Part model, mm, in its own coordinate system. Face numbers are marked on the shaded views. A direction names the side the tool comes from. Round coordinates to 2 decimals unless told otherwise and drop trailing zeros. Write each loop counter-clockwise with the first axis right and the second up, starting at its lowest first coordinate (ties: lowest second). Pieces come first, ordered by that corner, then holes. Notation, with made-up numbers: M -26,38 L 5,38 A29 ccw 5,67 Z; hole C -17.75,-2.5 d3. An arc over 180 degrees is marked long. Answer as a JSON object with one key per item and string values. Group by question number.
1. Two-plate mould, pull along X, no slides. Class the marked faces 1, 2 and 3: +X half, -X half, draft (parallel to the pull), parting line (faces both ways), or undercut.
2. Drop flat-ended pins along their axis: pin 1 (5 mm diameter, centred on y = 8, z = 6, fed in from +X); pin 2 (1.4 mm diameter, centred on x = -7, z = 15, fed in from +Y); pin 3 (1.8 mm diameter, centred on y = 11, z = 7.5, fed in from +X). Give the stop position or say it passes through.
3. Drill centre lines: line 1 (Z direction, x = -7.5, y = 2.55); line 2 (X direction, y = 5.25, z = 1.5); line 3 (Y direction, x = 5.75, z = 18.5). Where is each one in solid material? Low to high. Write a range as from..to.
4. Band-saw the part on D-D, the plane z = 16.25. Write the cut outline in (x, y).
5. Which spindle directions (+Z, -Z, +X, -X, +Y, -Y) get a long thin tool onto all of the face, cutting with end or side? Do the marked faces 4, 5 and 6. Say none if no direction does.
6. Band-saw the part on B-B, the plane z = 10. Write the cut outline in (x, y), plus the area to 3 significant figures.
7. Band-saw the part on C-C, the plane y = 2.5. Write the cut outline in (x, z), plus the area to 3 significant figures.
8. Band-saw the part on A-A, the plane x = -7.5. Write the cut outline in (y, z), plus the area to 3 significant figures.
from build123d import *

# Parameters (mm, degrees)
MAIN_DEPTH         = 20
SKETCH1_R          = 1.6
CUT_EXTRUDE1_DEPTH = 14


with BuildPart() as part:
    # Esquisse1 → Main (new body)
    with BuildSketch(Plane.XY):
        Polygon((-12.5, 0), (-12.5, 3), (-8.95, 3), (-8.95, 4), (-6.05, 4), (-6.05, 3), (-2.5, 3), (-2.5, 6.55), (-3.5, 6.55), (-3.5, 9.45), (-2.5, 9.45), (-2.5, 13), (0, 13), (0, 0), align=None)
    main = extrude(amount=MAIN_DEPTH)

    # Symétrie1: Main across plane
    add(main.mirror(Plane(origin=(0, 0, 0), x_dir=(0, 0, 1), z_dir=(1, 0, 0))))

    # Sketch1 → Cut-Extrude1 (cut, through all)
    with BuildSketch(Plane.XZ):
        with Locations((-7.5, 10)):
            Circle(SKETCH1_R)
        with Locations((7.5, 10)):
            Circle(SKETCH1_R)
    extrude(amount=-CUT_EXTRUDE1_DEPTH, mode=Mode.SUBTRACT)


solid = part.part
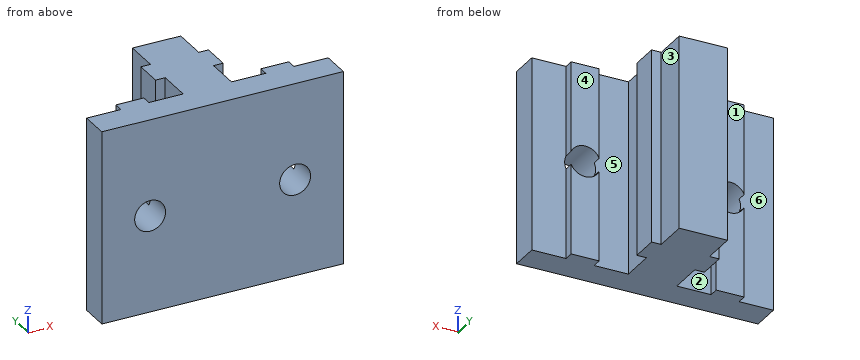
Worked answers:
{
 "1": {"face 1": "draft", "face 2": "undercut", "face 3": "+X half"},
 "2": {"pin 1": "stops at x = 3.5", "pin 2": "stops at y = 4", "pin 3": "stops at x = 2.5"},
 "3": {"line 1": "z = 0..8.4, 11.6..20", "line 2": "x = -2.5..2.5", "line 3": "y = 0..3"},
 "4": {"outline": "M -12.5,0 L 12.5,0 L 12.5,3 L 8.95,3 L 8.95,4 L 6.05,4 L 6.05,3 L 2.5,3 L 2.5,6.55 L 3.5,6.55 L 3.5,9.45 L 2.5,9.45 L 2.5,13 L -2.5,13 L -2.5,9.45 L -3.5,9.45 L -3.5,6.55 L -2.5,6.55 L -2.5,3 L -6.05,3 L -6.05,4 L -8.95,4 L -8.95,3 L -12.5,3 Z"},
 "5": {"face 4": "+Z, -Z, +X, +Y", "face 5": "+Z, -Z", "face 6": "+Z, -Z, -X, +Y"},
 "6": {"outline": "M -12.5,0 L -9.1,0 L -9.1,3 L -12.5,3 Z; M -5.9,0 L 5.9,0 L 5.9,3 L 2.5,3 L 2.5,6.55 L 3.5,6.55 L 3.5,9.45 L 2.5,9.45 L 2.5,13 L -2.5,13 L -2.5,9.45 L -3.5,9.45 L -3.5,6.55 L -2.5,6.55 L -2.5,3 L -5.9,3 Z; M 9.1,0 L 12.5,0 L 12.5,3 L 9.1,3 Z", "area": "112 mm^2"},
 "7": {"outline": "M -12.5,0 L 12.5,0 L 12.5,20 L -12.5,20 Z; hole C -7.5,10 d3.2; hole C 7.5,10 d3.2", "area": "484 mm^2"},
 "8": {"outline": "M 0,0 L 4,0 L 4,8.4 L 0,8.4 Z; M 0,11.6 L 4,11.6 L 4,20 L 0,20 Z", "area": "67.2 mm^2"}
}
